```python
from build123d import *

# Parameters (mm, degrees)
BOSS_EXTRUDE1_DEPTH = 1.68
SKETCH3_W           = 13.42
SKETCH3_H           = 12.62
BOSS_EXTRUDE2_DEPTH = 5.25
SKETCH4_R           = 3.45
BOSS_EXTRUDE3_DEPTH = 14.4
SKETCH5_W           = 44.4
SKETCH5_H           = 20.1
BOSS_EXTRUDE4_DEPTH = 1.6
SKETCH6_R           = 8
BOSS_EXTRUDE5_DEPTH = 12.4


with BuildPart() as part:
    # Sketch1 → Boss-Extrude1 (new body)
    with BuildSketch(Plane(origin=(0, 0, 0), x_dir=(1, 0, 0), z_dir=(0, 1, 0))):
        with BuildLine():
            Line((-42.5, 7.25), (42.5, 7.25))
            ThreePointArc((42.5, 7.25), (43.207106781, 6.957106781), (43.5, 6.25))
            Line((43.5, 6.25), (43.5, -6.25))
            ThreePointArc((43.5, -6.25), (43.207106781, -6.957106781), (42.5, -7.25))
            Line((42.5, -7.25), (-42.5, -7.25))
            ThreePointArc((-42.5, -7.25), (-43.207106781, -6.957106781), (-43.5, -6.25))
            Line((-43.5, -6.25), (-43.5, 6.25))
            ThreePointArc((-43.5, 6.25), (-43.207106781, 6.957106781), (-42.5, 7.25))
        make_face()
    extrude(amount=BOSS_EXTRUDE1_DEPTH)

    # Sketch3 → Boss-Extrude2 (add)
    with BuildSketch(Plane(origin=(0, 1.68, 0), x_dir=(1, 0, 0), z_dir=(0, 1, 0))):
        with Locations((28.19, 0)):
            Rectangle(SKETCH3_W, SKETCH3_H)
        with Locations((-28.19, 0)):
            Rectangle(SKETCH3_W, SKETCH3_H)
    extrude(amount=BOSS_EXTRUDE2_DEPTH)

    # Sketch4 → Boss-Extrude3 (add)
    with BuildSketch(Plane(origin=(0, 6.93, 0), x_dir=(1, 0, 0), z_dir=(0, 1, 0))):
        with Locations(Location((-28.19, 0, 0), (0, 0, 270))):
            Circle(SKETCH4_R)
        with Locations(Location((28.19, 0, 0), (0, 0, 90))):
            Circle(SKETCH4_R)
    extrude(amount=BOSS_EXTRUDE3_DEPTH)

    # Sketch5 → Boss-Extrude4 (add)
    with BuildSketch(Plane.XY.offset(7.25)):
        with Locations((0, -10.05)):
            Rectangle(SKETCH5_W, SKETCH5_H)
    extrude(amount=-BOSS_EXTRUDE4_DEPTH)

    # Sketch6 → Boss-Extrude5 (add)
    with BuildSketch(Plane.XY.offset(7.25)):
        with Locations(Location((11.1, -10.05, 0), (0, 0, 180))):
            Circle(SKETCH6_R)
        with Locations(Location((-11.1, -10.05, 0), (0, 0, 180))):
            Circle(SKETCH6_R)
    extrude(amount=BOSS_EXTRUDE5_DEPTH)


solid = part.part
```
Work out the finished part from the listing and answer in its coordinate system (mm). A direction names the side the tool comes from. Give positions to 0.01 mm unless a question says otherwise; leave off trailing zeros. Loops run counter-clockwise (first coordinate to the right, second up) from the corner with the lowest first, then second, coordinate; pieces in that order, holes last. Notation, with made-up numbers: (-37, 29.5) -> (-8, 29.5) arc R20 ccw to (-8, 59.5) -> close; hole circle Ø10 at (32, 70). An arc over 180 degrees is marked (long way). Put each result on its own line as item: value. Start each with the question number.
Item 1: The part is cut by section B-B (z = 0). Give the vertices of the cut face in (x, y), then the cut area to 3 significant figures.
Item 2: Find the intervals of material crossed by L1, parallel to X at y = -10, z = 7.5; L2, parallel to Y at x = -3.5, z = -0.25; L3, parallel to Z at x = 34.5, y = 6, in increasing order. Write a range as [from, to].
Item 3: The part is cut by section D-D (y = -10.05). Give the vertices of the cut face in (x, z), then the cut area to 3 significant figures.
Item 4: The mould has two halves that part along X. Classify faces 6 (the face through (-24.77, 14.03, -0.45)), 7 (the face through (-28, 4, -6.31)), 8 (the face through (43.5, 1, 0)): released by +X, released by -X, zero draft, split by the parting line, or undercut.
Item 5: Each of these flat-tipped pins is pushed along its axis until it touches: P1, Ø6, axis at x = -29.5, y = 5.5, coming from the -Z side; P2, Ø4, axis at x = -16, z = 16.5, coming from the +Y side; P3, Ø0.5, axis at y = -15, z = 6.5, coming from the -X side. Where does it stop, or does it pass through?
Item 6: Which of the six approach directions +Z, -Z, +X, -X, +Y, -Y give full straight-line access (tool end or side, diameter ignored) to faces 1 (the face through (-34.9, 4, 0)), 2 (the face through (19.092, -10.402, 13.363)), 3 (the face through (-28, 4, 6.31)), 4 (the face through (34.9, 4, 0)), 5 (the face through (0, -10, 5.65))?
Item 7: The part is cut by section C-C (z = 15.75). Give the vertices of the cut face in (x, y).
Item 8: The part is cut by section A-A (x = -28.19). Give the vertices of the cut face in (y, z).
Answers below:
1. outline: (-43.5, 0) -> (43.5, 0) -> (43.5, 1.68) -> (34.9, 1.68) -> (34.9, 6.93) -> (31.64, 6.93) -> (31.64, 21.33) -> (24.74, 21.33) -> (24.74, 6.93) -> (21.48, 6.93) -> (21.48, 1.68) -> (-21.48, 1.68) -> (-21.48, 6.93) -> (-24.74, 6.93) -> (-24.74, 21.33) -> (-31.64, 21.33) -> (-31.64, 6.93) -> (-34.9, 6.93) -> (-34.9, 1.68) -> (-43.5, 1.68) -> close
1. area: 486 mm2
2. L1: [-19.1, -3.1], [3.1, 19.1]
2. L2: [0, 1.68]
2. L3: [-6.31, 6.31]
3. outline: (-22.2, 5.65) -> (22.2, 5.65) -> (22.2, 7.25) -> (19.1, 7.25) -> (19.1, 19.65) -> (3.1, 19.65) -> (3.1, 7.25) -> (-3.1, 7.25) -> (-3.1, 19.65) -> (-19.1, 19.65) -> (-19.1, 7.25) -> (-22.2, 7.25) -> close
3. area: 468 mm2
4. face 6: undercut
4. face 7: zero draft
4. face 8: released by +X
5. P1: z = -6.31
5. P2: y = -2.59
5. P3: x = -22.2
6. face 1: +Z, -Z, -X, +Y
6. face 2: +Z
6. face 3: +Z, +X, -X, +Y
6. face 4: +Z, -Z, +X, +Y
6. face 5: -Z, +X, -X, -Y
7. outline: circle Ø16 at (-11.1, -10.05); circle Ø16 at (11.1, -10.05)
8. outline: (0, -7.25) -> (1.68, -7.25) -> (1.68, -6.31) -> (6.93, -6.31) -> (6.93, -3.45) -> (21.33, -3.45) -> (21.33, 3.45) -> (6.93, 3.45) -> (6.93, 6.31) -> (1.68, 6.31) -> (1.68, 7.25) -> (0, 7.25) -> close
